from build123d import *

# Parameters (mm, degrees)
SKETCH1_W                            = 660
SKETCH1_H                            = 3
PACK_KALIP_PLAKASI_3MM_66X79_1_DEPTH = 790
PACK_KALIP_PLAKASI_3MM_66X79_2_START = -237.5
SKETCH2_W                            = 325
SKETCH2_H                            = 5
PACK_KALIP_PLAKASI_3MM_66X79_2_DEPTH = 325


with BuildPart() as part:
    # Sketch1 → PACK_kalip_plakasi_3mm_66x79_1 (new body)
    with BuildSketch(Plane.XY):
        with Locations((350, 598.5)):
            Rectangle(SKETCH1_W, SKETCH1_H)
    extrude(amount=-PACK_KALIP_PLAKASI_3MM_66X79_1_DEPTH)

    # Sketch2 → PACK_kalip_plakasi_3mm_66x79_2 (cut)
    with BuildSketch(Plane.XY.offset(PACK_KALIP_PLAKASI_3MM_66X79_2_START)):
        with Locations((350, 598.5)):
            Rectangle(SKETCH2_W, SKETCH2_H)
    extrude(amount=-PACK_KALIP_PLAKASI_3MM_66X79_2_DEPTH, mode=Mode.SUBTRACT)


solid = part.part
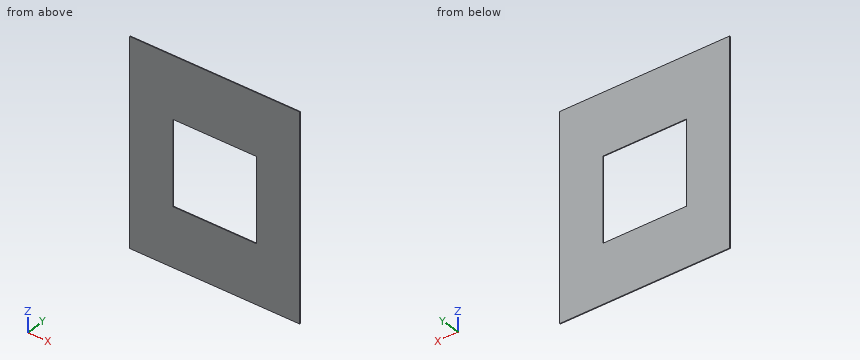
Model file for the job. Use its own axes, mm. Coordinates: 2 decimals unless noted, no trailing zeros. Order: outer loops, then holes, each group sorted by start corner. A loop starts at its lowest first (then second) coordinate and runs counter-clockwise, first axis right, second up. Notation, with made-up numbers: (80, -39) -> (105, -39) arc R27 ccw to (105, -3) -> close; hole circle Ø3 at (30.25, 41). An arc over 180 degrees is marked (long way). Return JSON: item names as keys, results as strings. Group by question number.
Item 1: Saw through at A-A on y = 598.5. Write the cut outline in (x, z), then the cut area to 3 significant figures.
Item 2: Wall check: line 1 along X through (y, z) = (598, -385); line 2 along Z through (x, y) = (241, 599.25). Give the ranges that are in metal, low to high. Write a range as [from, to].
Item 3: Saw through at C-C on x = 365. Write the cut outline in (y, z).
Item 4: Saw through at B-B on z = -331. Write the cut outline in (x, y).
Values found:
{
 "1": {"outline": "(20, -790) -> (680, -790) -> (680, 0) -> (20, 0) -> close; hole (187.5, -562.5) -> (512.5, -562.5) -> (512.5, -237.5) -> (187.5, -237.5) -> close", "area": "416,000 mm2"},
 "2": {"line 1": "x = [20, 187.5], [512.5, 680]", "line 2": "z = [-790, -562.5], [-237.5, 0]"},
 "3": {"outline": "(597, -790) -> (600, -790) -> (600, -562.5) -> (597, -562.5) -> close; (597, -237.5) -> (600, -237.5) -> (600, 0) -> (597, 0) -> close"},
 "4": {"outline": "(20, 597) -> (187.5, 597) -> (187.5, 600) -> (20, 600) -> close; (512.5, 597) -> (680, 597) -> (680, 600) -> (512.5, 600) -> close"}
}
